For this review, use the dimensioned drawing (mm, ordinates from the lowest corner) and the shaded views. Round coordinates to 2 decimals unless told otherwise and drop trailing zeros. Loops run counter-clockwise (first coordinate to the right, second up) from the corner with the lowest first, then second, coordinate; pieces in that order, holes last. Notation, with made-up numbers: M 0.25,89.25 L 27.25,89.25 A18 ccw 27.25,93.25 Z; hole C 22,88.25 d10. An arc over 180 degrees is marked long. Answer as a JSON object with one key per item and string values. Group by question number.
Item 1: Consider section D-D (z = 30.5). Give the boundary of the cut face in (x, y).
Item 2: Consider section A-A (x = 13). Give the boundary of the cut face in (y, z), and give its area (3 significant figures).
Item 3: Consider section C-C (y = 2.75). State how many separate pieces and enclosed holes the cut face has, and give its area (3 significant figures).
Item 4: Consider section B-B (z = 22.5). Give the boundary of the cut face in (x, y).
Item 5: Insertion check: P1, Ø1, axis at x = 17, y = 2, coming from the -Z side; P2, Ø3, axis at x = 21.5, y = 7, coming from the -Z side; P3, Ø3, axis at y = 5, z = 19, coming from the -X side. Each pin has a flat end and moves straight along its axis. Give the tip position at first contact, or say it passes through.
Item 6: To check wall thickness, follow line 1 (X direction, y = 3.5, z = 22); line 2 (X direction, y = 3.5, z = 23); line 3 (X direction, y = 1.25, z = 6.5). State the ranges of each line that lie inside material, in increasing order.
Item 7: The part is to be moulded in two halves that separate along X. For the marked faces 1, 2 and 3, say which applies: +X half, -X half, draft (parallel to the pull), parting line (faces both ways), or undercut.
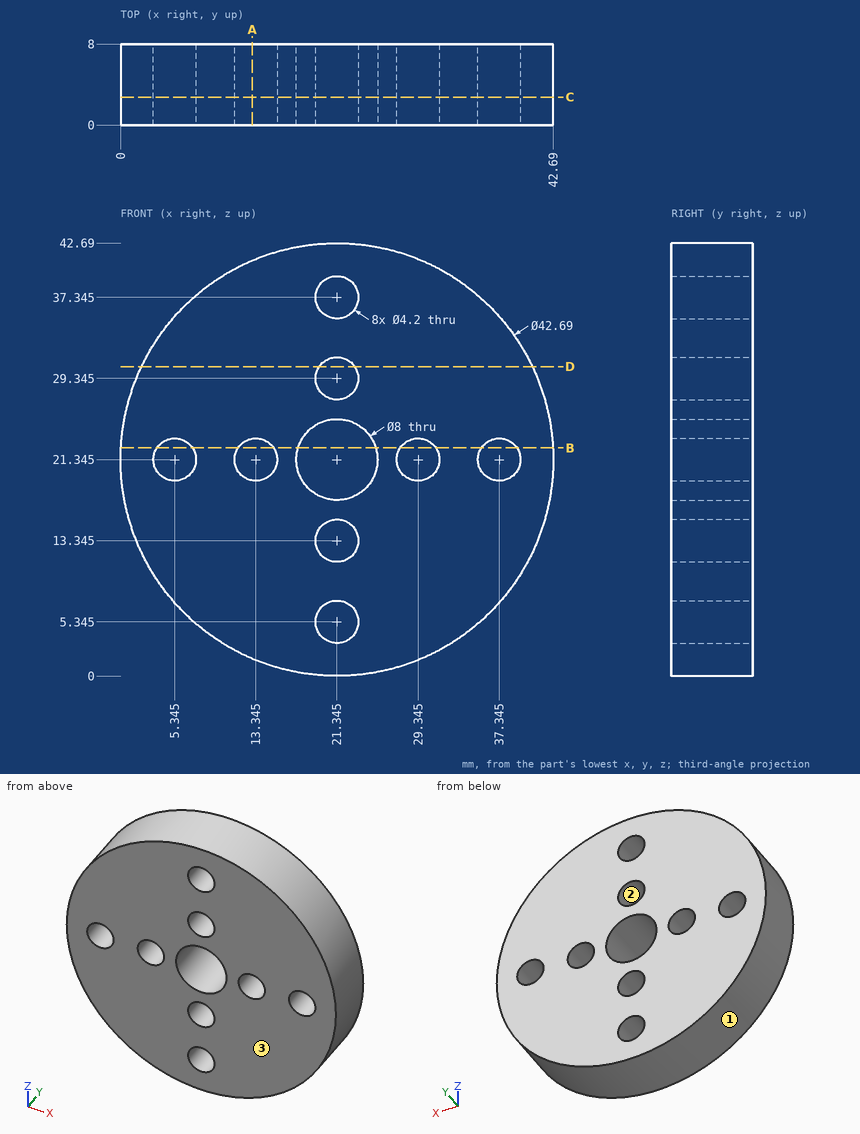
Geometry results:
{
 "1": {"outline": "M 2.06,0 L 19.59,0 L 19.59,8 L 2.06,8 Z; M 23.1,0 L 40.63,0 L 40.63,8 L 23.1,8 Z"},
 "2": {"outline": "M 0,1.7 L 8,1.7 L 8,19.27 L 0,19.27 Z; M 0,23.42 L 8,23.42 L 8,40.99 L 0,40.99 Z", "area": "281 mm^2"},
 "3": {"separate pieces": "1", "enclosed holes": "9", "area": "1,270 mm^2"},
 "4": {"outline": "M 0.03,0 L 3.59,0 L 3.59,8 L 0.03,8 Z; M 7.1,0 L 11.59,0 L 11.59,8 L 7.1,8 Z; M 15.1,0 L 17.52,0 L 17.52,8 L 15.1,8 Z; M 25.17,0 L 27.59,0 L 27.59,8 L 25.17,8 Z; M 31.1,0 L 35.59,0 L 35.59,8 L 31.1,8 Z; M 39.1,0 L 42.66,0 L 42.66,8 L 39.1,8 Z"},
 "5": {"P1": "stops at z = 0.35", "P2": "stops at z = 0", "P3": "stops at x = 0.02"},
 "6": {"line 1": "x = 0.01 to 3.35, 7.34 to 11.35, 15.34 to 17.4, 25.29 to 27.35, 31.34 to 35.35, 39.34 to 42.68", "line 2": "x = 0.06 to 4.05, 6.64 to 12.05, 14.64 to 17.7, 24.99 to 28.05, 30.64 to 36.05, 38.64 to 42.63", "line 3": "x = 6.01 to 19.59, 23.1 to 36.68"},
 "7": {"face 1": "parting line", "face 2": "undercut", "face 3": "draft"}
}
